```python
from build123d import *

# Parameters (mm, degrees)
F1_DEPTH      = 19.05
F2_R          = 9.525
F3_R          = 5.08
F5_DEPTH      = 3.175
F5_DEPTH_BACK = 5.08
F6_R          = 2.54
F7_R          = 4.7625
F8_DEPTH      = 19.05
F9_SIZE       = 0.762


with BuildPart() as f1:
    # F0 (on Front) → F1 (new body)
    with BuildSketch(Plane.XZ):
        with BuildLine():
            Line((71.9126091726, 0), (71.9126091726, 38.1))
            ThreePointArc((71.9126091726, 38.1), (8.4126091726, 44.7879573046), (-55.0873908274, 38.1))
            Line((-55.0873908274, 38.1), (-55.0873908274, 0))
            Line((-55.0873908274, 0), (-55.0873908274, -38.1))
            ThreePointArc((-55.0873908274, -38.1), (8.4126091726, -44.7879573046), (71.9126091726, -38.1))
            Line((71.9126091726, -38.1), (71.9126091726, 0))
        make_face()
    extrude(amount=F1_DEPTH)

    # F2
    f2_edges = [f1.edges().sort_by_distance(p)[0] for p in [
        (-55.087391, -9.525, 38.1),
        (-55.087391, -9.525, -38.1),
        (71.912609, -9.525, 38.1),
        (71.912609, -9.525, -38.1),
    ]]
    fillet(f2_edges, radius=F2_R)

    # F3
    f3_edges = [f1.edges().sort_by_distance(p)[0] for p in [
        (8.412609, -19.05, 44.787957),
        (8.412609, 0, 44.787957),
    ]]
    fillet(f3_edges, radius=F3_R)

    # F4 (on face) → F5 (join, two sides)
    with BuildSketch(Plane(origin=(-55.0873908274, 0, 0), x_dir=(0, -1, 0), z_dir=(-1, 0, 0))) as f5_sk:
        with BuildLine():
            ThreePointArc((13.97, -4.9615211664), (15.7291776693, -2.7529165008), (16.3569446489, 0))
            ThreePointArc((16.3569446489, 0), (15.7291776693, 2.7529165008), (13.97, 4.9615211664))
            Line((13.97, 4.9615211664), (13.97, -4.9615211664))
        make_face()
        with BuildLine():
            Line((5.08, -4.0059601129), (5.08, 4.0059601129))
            ThreePointArc((5.08, 4.0059601129), (3.6569446489, 0), (5.08, -4.0059601129))
        make_face()
        with BuildLine():
            Line((13.97, -4.9615211664), (13.97, 4.9615211664))
            ThreePointArc((13.97, 4.9615211664), (9.3283100813, 6.3136324825), (5.08, 4.0059601129))
            Line((5.08, 4.0059601129), (5.08, -4.0059601129))
            ThreePointArc((5.08, -4.0059601129), (9.3283100813, -6.3136324825), (13.97, -4.9615211664))
        make_face()
    extrude(amount=F5_DEPTH)
    extrude(f5_sk.sketch, amount=-F5_DEPTH_BACK)

    # F6
    f6_edges = [f1.edges().sort_by_distance(p)[0] for p in [
        (-58.262391, -6.043889, -4.961521),
    ]]
    fillet(f6_edges, radius=F6_R)

    # F7 (on face) → F8 (join)
    with BuildSketch(Plane(origin=(-58.2623908274, 0, 0), x_dir=(0, -1, 0), z_dir=(-1, 0, 0))):
        with Locations((10.0069446489, 0)):
            Circle(F7_R)
    extrude(amount=F8_DEPTH)

    # F9
    f9_edges = [f1.edges().sort_by_distance(p)[0] for p in [
        (-77.312391, -5.244445, 0),
    ]]
    chamfer(f9_edges, length=F9_SIZE)


solid = f1.part
```
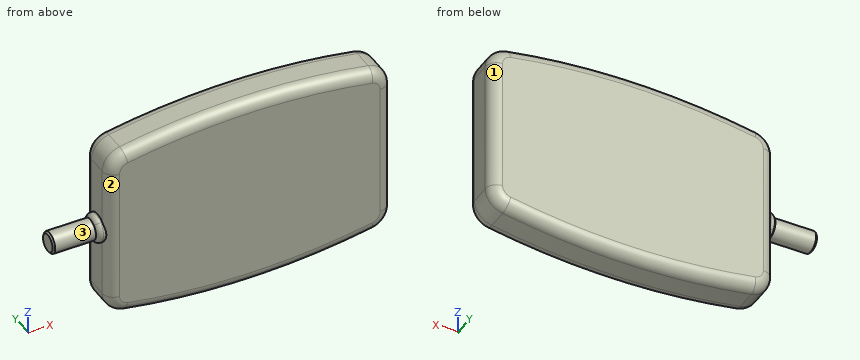
For this review, take the finished solid that the model builds, in its own axes (mm). Face numbers are marked on the shaded views. A direction names the side the tool comes from. Coordinates: 2 decimals unless noted, no trailing zeros. Order: outer loops, then holes, each group sorted by start corner. A loop starts at its lowest first (then second) coordinate and runs counter-clockwise, first axis right, second up. Notation, with made-up numbers: (-16, 65) - (8, 65) arc R28 ccw to (8, 93) - close; hole circle Ø1 at (2, 6). An arc over 180 degrees is marked (long way). Answer as a JSON object with one key per item and string values. Group by question number.
1. For probe 1 along X at (y, z) = (-6.75, 8.5); probe 2 along Z at (x, y) = (-33.5, -14.75); probe 3 along X at (y, z) = (-18.25, 24.5), list the stretches that pass through material, from the lowest coordinate up.
2. For the marked faces 1, 2 and 3, list the 3-axis set-ups (+Z, -Z, +X, -X, +Y, -Y) from which the entire face can be reached by the end or side of a thin tool; tool diameter is ignored.
3. Clearance check with flat-ended pins moving along their axes: P1, Ø2.5, axis at y = -7.5, z = 12.5, coming from the -X side; P2, Ø10, axis at x = -6, y = -9, coming from the +Z side; P3, Ø4, axis at x = 24.5, y = -16.5, coming from the -Z side. State where each tip first meets the part, or that it passes through.
4. We need section A-A on z = 14.5. State the section outline as (x, y) points, then the cut area to 3 significant figures.
Final values:
{
 "1": {"probe 1": "-55.09 to 71.91", "probe 2": "-41.83 to 41.83", "probe 3": "-52.74 to 69.57"},
 "2": {"face 1": "+Z, -Z, +X, +Y", "face 2": "-X, -Y", "face 3": "-X"},
 "3": {"P1": "x = -55.09", "P2": "z = 44.64", "P3": "z = -44.36"},
 "4": {"outline": "(-55.09, -13.97) arc R5.08 ccw to (-50.01, -19.05) - (66.83, -19.05) arc R5.08 ccw to (71.91, -13.97) - (71.91, -5.08) arc R5.08 ccw to (66.83, 0) - (-50.01, 0) arc R5.08 ccw to (-55.09, -5.08) - close", "area": "2,400 mm²"}
}
